from build123d import *


with BuildPart() as f2:
    # F2: sweep along a path in F0
    with BuildLine(Plane.XY) as f2_path:
        Line((70, -38.6713670124), (70, 42.1394666243))
        ThreePointArc((70, 42.1394666243), (67.7082039325, 49.1928896518), (61.7082039325, 53.5521448199))
        Line((61.7082039325, 53.5521448199), (-18.44582472, 79.5957674615))
        ThreePointArc((-18.44582472, 79.5957674615), (-25.862232585, 79.5957674615), (-31.862232585, 75.2365122934))
        Line((-31.862232585, 75.2365122934), (-81.4001466275, 7.0534230275))
        ThreePointArc((-81.4001466275, 7.0534230275), (-83.691942695, 0), (-81.4001466275, -7.0534230275))
        Line((-81.4001466275, -7.0534230275), (-31.862232585, -75.2365122934))
        ThreePointArc((-31.862232585, -75.2365122934), (-25.862232585, -79.5957674615), (-18.44582472, -79.5957674615))
        Line((-18.44582472, -79.5957674615), (57.5640973422, -54.8986466743))
    # F1 (on Front) → F2 (sweep)
    with BuildSketch(Plane.XZ):
        Polygon((61, -2.5), (79, -2.5), (79, 2.5), (77, 2.5), (77, 1.5), (75, 1.5), (75, 2.5), (65, 2.5), (65, 1.5), (63, 1.5), (63, 2.5), (61, 2.5), align=None)
    sweep(path=f2_path.line)


solid = f2.part
Geometry check sheet. Reference: the model listing, model coordinates, mm. A direction names the side the tool comes from. Coordinates: 2 decimals unless noted, no trailing zeros. Order: outer loops, then holes, each group sorted by start corner. A loop starts at its lowest first (then second) coordinate and runs counter-clockwise, first axis right, second up. Notation, with made-up numbers: (66.5, -27.5) - (74.5, -27.5) arc R22 cw to (74.5, -0.5) - close; hole circle Ø10 at (-13.5, 87.5). An arc over 180 degrees is marked (long way). Answer in a Markdown table with one row per item. Add a question column.
1) Cross-section at C-C, the plane z = 0. Record the cut outline in (x, y).
2) Release check for a two-part mould opening along Y. For faces 4 (the flat face through (61, 2, 0)), 5 (the flat face through (22.254, -73.732, 2.007)), 6 (the cylindrical face through (75.1, 54.33, 0.04)) record: +Y half, -Y half, draft (parallel to the pull), parting line (faces both ways), or undercut.
3) Cross-section at B-B, the plane x = 14. Record the cut outline in (y, z), then the cut area to 3 significant figures.
4) Gauge pin test, flat end, axial feed: P1, Ø1.5, axis at y = 47, z = -1, coming from the -X side. Record the tip position at first contact, or that the pin passes through.
5) Material ranges on line 1 along X through (y, z) = (32, 1.8); line 2 along Y through (x, z) = (-84.5, 2.35); line 3 along X through (y, z) = (22, 2.2), recorded low to high. Write a range as [from, to].
6) Cross-section at A-A, the plane y = 34. Record the cut outline in (x, z), then the cut area to 3 significant figures.
7) Set-up check for faces 1 (the flat face through (-49.697, 35.378, 0.035)), 2 (the flat face through (-52.93, 37.73, 2.01)), 3 (the flat face through (79, 2, 0)): record each of +Z, -Z, +X, -X, +Y, -Y from which the full face is reachable in a straight line by a thin tool's end or side.
8) Cross-section at D-D, the plane x = 67. Record the cut outline in (y, z), then the cut area to 3 significant figures.
Check result:
| question | item | result |
|---|---|---|
| 1 | outline | (-88.68, -12.34) - (-39.14, -80.53) arc R21 ccw to (-15.66, -88.16) - (60.35, -63.46) - (54.78, -46.34) - (-21.23, -71.04) arc R3 cw to (-24.58, -69.95) - (-74.12, -1.76) arc R3 cw to (-74.12, 1.76) - (-24.58, 69.95) arc R3 cw to (-21.23, 71.04) - (58.93, 44.99) arc R3 cw to (61, 42.14) - (61, -38.67) - (79, -38.67) - (79, 42.14) arc R21 ccw to (64.49, 62.11) - (-15.66, 88.16) arc R21 ccw to (-39.14, 80.53) - (-88.68, 12.34) arc R21 ccw to start |
| 2 | face 4 | draft |
| 2 | face 5 | undercut |
| 2 | face 6 | +Y half |
| 3 | outline | (-78.52, -2.5) - (-59.59, -2.5) - (-59.59, 2.5) - (-61.69, 2.5) - (-61.69, 1.5) - (-63.8, 1.5) - (-63.8, 2.5) - (-74.31, 2.5) - (-74.31, 1.5) - (-76.41, 1.5) - (-76.41, 2.5) - (-78.52, 2.5) - close; (59.59, -2.5) - (78.52, -2.5) - (78.52, 2.5) - (76.41, 2.5) - (76.41, 1.5) - (74.31, 1.5) - (74.31, 2.5) - (63.8, 2.5) - (63.8, 1.5) - (61.69, 1.5) - (61.69, 2.5) - (59.59, 2.5) - close |
| 3 | area | 181 mm² |
| 4 | P1 | stops at x = -64.05 |
| 5 | line 1 | x = [-74.4, -71.93], [-69.46, -57.1], [-54.62, -52.15], [61, 63], [65, 75], [77, 79] |
| 5 | line 2 | y = [-18.1, -14.7], [-11.29, 11.29], [14.7, 18.1] |
| 5 | line 3 | x = [-81.67, -79.19], [-76.72, -64.36], [-61.89, -59.42], [61, 63], [65, 75], [77, 79] |
| 6 | outline | (-72.95, -2.5) - (-50.7, -2.5) - (-50.7, 2.5) - (-53.17, 2.5) - (-53.17, 1.5) - (-55.64, 1.5) - (-55.64, 2.5) - (-68, 2.5) - (-68, 1.5) - (-70.47, 1.5) - (-70.47, 2.5) - (-72.95, 2.5) - close; (61, -2.5) - (79, -2.5) - (79, 2.5) - (77, 2.5) - (77, 1.5) - (75, 1.5) - (75, 2.5) - (65, 2.5) - (65, 1.5) - (63, 1.5) - (63, 2.5) - (61, 2.5) - close |
| 6 | area | 192 mm² |
| 7 | face 1 | +Z, -Z |
| 7 | face 2 | +Z |
| 7 | face 3 | +Z, -Z, +X, +Y, -Y |
| 8 | outline | (-38.67, -2.5) - (61.11, -2.5) - (61.11, 2.5) - (58.87, 2.5) - (58.87, 1.5) - (56.56, 1.5) - (56.56, 2.5) - (-38.67, 2.5) - close |
| 8 | area | 497 mm² |
